```python
from build123d import *

# Parameters (mm, degrees)
SKETCH1_R           = 40
SKETCH1_R_2         = 35
BOSS_EXTRUDE1_DEPTH = 30
SKETCH2_W           = 120
SKETCH2_H           = 100
BOSS_EXTRUDE2_DEPTH = 10
FILLET4_R           = 10
FILLET5_R           = 10


with BuildPart() as part:
    # Sketch1 → Boss-Extrude1 (new body)
    with BuildSketch(Plane(origin=(0, 0, 0), x_dir=(1, 0, 0), z_dir=(0, 1, 0))):
        with Locations(Location((0, 0, 0), (0, 0, 270))):
            Circle(SKETCH1_R)
        with Locations(Location((0, 0, 0), (0, 0, 270))):
            Circle(SKETCH1_R_2, mode=Mode.SUBTRACT)
    extrude(amount=BOSS_EXTRUDE1_DEPTH)

    # Sketch2 → Boss-Extrude2 (add)
    with BuildSketch(Plane.XZ):
        Rectangle(SKETCH2_W, SKETCH2_H)
    extrude(amount=BOSS_EXTRUDE2_DEPTH)

    # Fillet4
    fillet4_edges = [part.edges().sort_by_distance(p)[0] for p in [
        (60, -5, -50),
        (60, -5, 50),
        (-60, -5, 50),
        (-60, -5, -50),
    ]]
    fillet(fillet4_edges, radius=FILLET4_R)

    # Fillet5
    fillet5_edges = [part.edges().sort_by_distance(p)[0] for p in [
        (57.071067812, 0, -47.071067812),
        (0, 0, -50),
        (-57.071067812, 0, -47.071067812),
        (-60, 0, 0),
        (-57.071067812, 0, 47.071067812),
        (0, 0, 50),
        (57.071067812, 0, 47.071067812),
        (60, 0, 0),
    ]]
    fillet(fillet5_edges, radius=FILLET5_R - 0.0001)  # a hair under: the kernel refuses the full size


solid = part.part
```
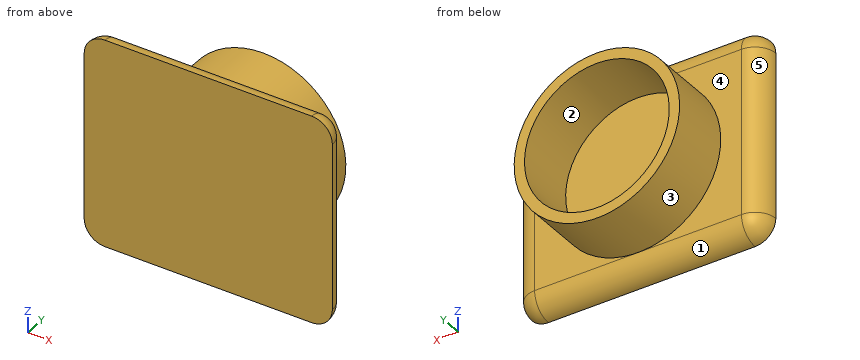
CAD build for the part. Positions are in the model's coordinates, mm. Face numbers are marked on the shaded views. A direction names the side the tool comes from. Round coordinates to 2 decimals unless told otherwise and drop trailing zeros. Order: outer loops, then holes, each group sorted by start corner. A loop starts at its lowest first (then second) coordinate and runs counter-clockwise, first axis right, second up. Notation, with made-up numbers: (18.25, -7) - (28.25, -7) arc R33 cw to (28.25, 25) - close; hole circle Ø11 at (74, -4.75). An arc over 180 degrees is marked (long way). Answer in a Markdown table with one row per item. Add a question column.
(1) 3-axis set-ups, long thin cutter, end or side, ignore diameter. For the marked faces 4 and 5: which of +Z, -Z, +X, -X, +Y, -Y reach the whole face in a straight line?
(2) Drop flat-ended pins along their axis: pin 1 Ø1 at (y, z) = (12.5, -10) entering from +X; pin 2 Ø4 at (x, y) = (-29, 24) entering from -Z; pin 3 Ø4 at (x, y) = (14, -5.5) entering from -Z. Give the stop position or say it passes through.
(3) Mould opens along Z. For the marked faces 1, 2 and 3 say: +Z half, -Z half, draft (parallel to the pull), parting line (faces both ways), or undercut.
(4) Band-saw the part on C-C on y = 12. List the corners of the cut face in (x, z).
(5) Probe L1, parallel to X at y = 17.25, z = 0; L2, parallel to Y at x = -8, z = 4.5; L3, parallel to Z at x = 29, y = 13. List the from-to ranges inside material, lowest first. Write a range as [from, to].
Data:
| question | item | result |
|---|---|---|
| 1 | face 4 | +Y |
| 1 | face 5 | +Z, -Z, -X, +Y |
| 2 | pin 1 | stops at x = 38.86 |
| 2 | pin 2 | stops at z = -29.51 |
| 2 | pin 3 | stops at z = -49.68 |
| 3 | face 1 | -Z half |
| 3 | face 2 | undercut |
| 3 | face 3 | parting line |
| 4 | outline | circle Ø80 at (0, 0); hole circle Ø70 at (0, 0) |
| 5 | L1 | x = [-40, -35], [35, 40] |
| 5 | L2 | y = [-10, 0] |
| 5 | L3 | z = [-27.55, -19.6], [19.6, 27.55] |
